Geometry check sheet. Reference: drawing and pictorial views, mm from the part's lowest x, y, z. Give positions to 0.01 mm unless a question says otherwise; leave off trailing zeros. Order: outer loops, then holes, each group sorted by start corner. A loop starts at its lowest first (then second) coordinate and runs counter-clockwise, first axis right, second up.
Item 1: Sectioned sample at D-D on z = 31. Record the boundary of the cut face in (x, y).
Item 2: Gauge pin test, flat ends, axial feed: P1, Ø2.5, axis at x = 89, y = 6.5, coming from the +Z side; P2, Ø5, axis at x = 23.5, z = 19.5, coming from the +Y side; P3, Ø2.5, axis at x = 95, y = 5, coming from the -Z side; P4, Ø3, axis at x = 57.5, y = 5.5, coming from the +Z side. Record the tip position at first contact, or that the pin passes through.
Item 3: Sectioned sample at B-B on z = 39. Record the boundary of the cut face in (x, y), and give its area (3 significant figures).
Item 4: Material ranges on line 1 along Z through (x, y) = (93.5, 6.75); line 2 along X through (y, z) = (5.75, 7); line 3 along X through (y, z) = (7.75, 3.5), recorded low to high.
Item 5: Sectioned sample at C-C on x = 88. Record the boundary of the cut face in (y, z), and give its area (3 significant figures).
Item 6: Sectioned sample at A-A on y = 4.75. Record the boundary of the cut face in (x, z), and give its area (3 significant figures).
Item 7: Release check for a two-part mould opening along X. For the marked faces 1 and 2 record: released by +X, released by -X, zero draft, split by the parting line, or undercut.
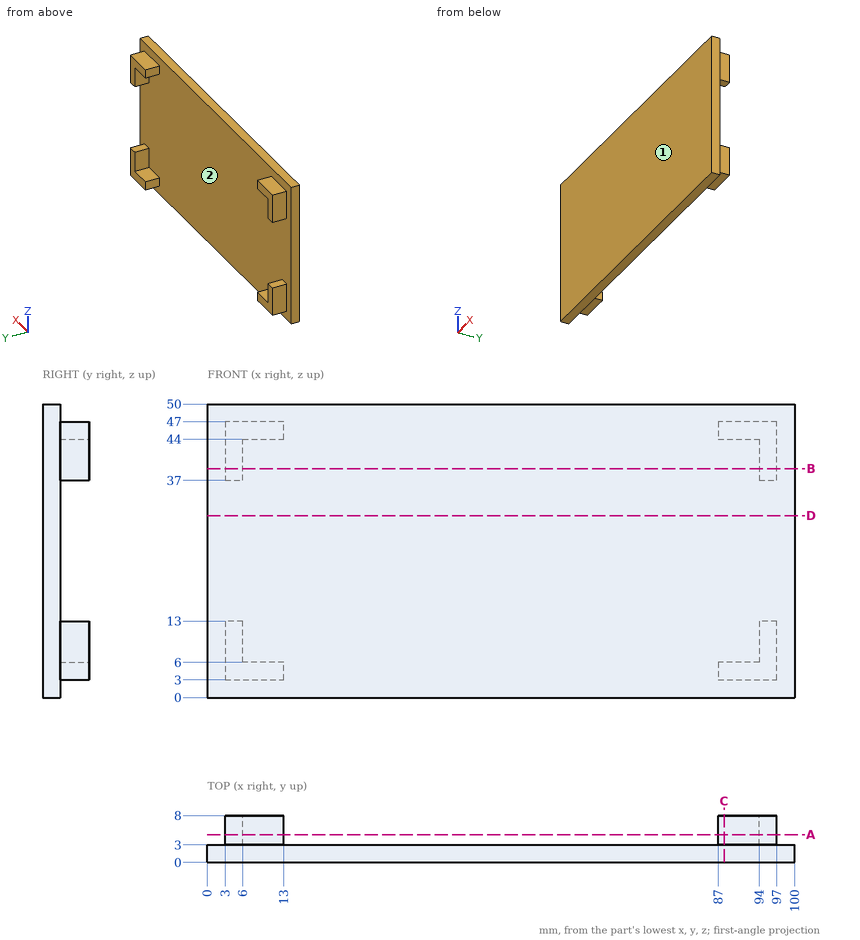
Report:
1. outline: (0, 0) - (100, 0) - (100, 3) - (0, 3) - close
2. P1: stops at z = 47
2. P2: stops at y = 3
2. P3: stops at z = 3
2. P4: passes through
3. outline: (0, 0) - (100, 0) - (100, 3) - (97, 3) - (97, 8) - (94, 8) - (94, 3) - (6, 3) - (6, 8) - (3, 8) - (3, 3) - (0, 3) - close
3. area: 330 mm2
4. line 1: z = 3 to 6, 44 to 47
4. line 2: x = 3 to 6, 94 to 97
4. line 3: x = 3 to 13, 87 to 97
5. outline: (0, 0) - (3, 0) - (3, 3) - (8, 3) - (8, 6) - (3, 6) - (3, 44) - (8, 44) - (8, 47) - (3, 47) - (3, 50) - (0, 50) - close
5. area: 180 mm2
6. outline: (3, 3) - (13, 3) - (13, 6) - (6, 6) - (6, 13) - (3, 13) - close; (3, 37) - (6, 37) - (6, 44) - (13, 44) - (13, 47) - (3, 47) - close; (87, 3) - (97, 3) - (97, 13) - (94, 13) - (94, 6) - (87, 6) - close; (87, 44) - (94, 44) - (94, 37) - (97, 37) - (97, 47) - (87, 47) - close
6. area: 204 mm2
7. face 1: zero draft
7. face 2: undercut
